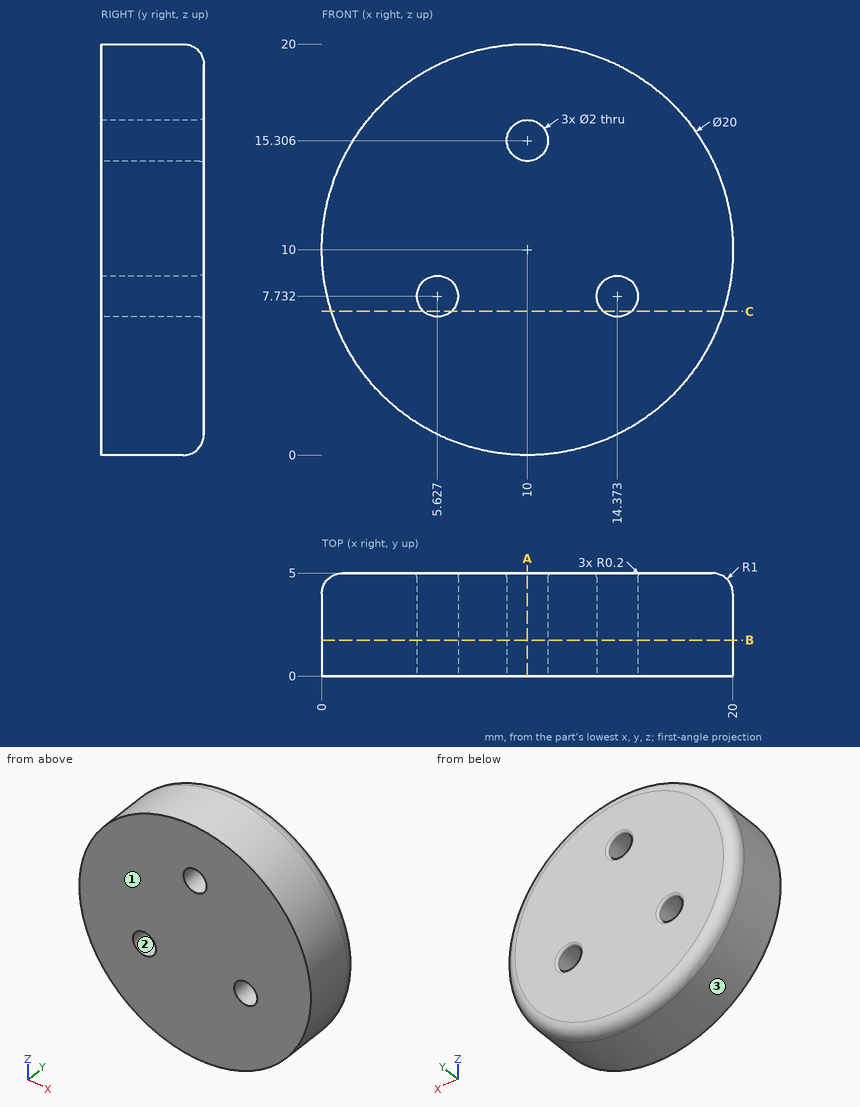
Job drawing, mm, ordinate dimensions from the low corner. One solid piece. Coordinates: 2 decimals unless noted, no trailing zeros. Order: outer loops, then holes, each group sorted by start corner. A loop starts at its lowest first (then second) coordinate and runs counter-clockwise, first axis right, second up. Notation, with made-up numbers: (1.5, -38) - (19.5, -38) arc R27 cw to (19.5, -7) - close; hole circle Ø8 at (-26, -5). An arc over 180 degrees is marked (long way). Write each question's results on one line, items separated by ' | '. Start each with the question number.
Item 1: Wall check: probe 1 along X at (y, z) = (4.5, 15.25); probe 2 along X at (y, z) = (0.6, 10); probe 3 along Z at (x, y) = (3, 1). Give the ranges that are in metal, low to high. Write a range as [from, to].
Item 2: Band-saw the part on B-B on y = 1.75. Write the cut outline in (x, z), and give its area (3 significant figures).
Item 3: Band-saw the part on A-A on x = 10. Write the cut outline in (y, z).
Item 4: Flat gauge pins, fed straight in: pin 1 (1 mm diameter, centred on y = 4, z = 2.5, fed in from +X); pin 2 (1 mm diameter, centred on x = 3.5, y = 3, fed in from +Z); pin 3 (2 mm diameter, centred on x = 2, y = 2, fed in from +Z). Where does each tip first touch, or does it go through?
Item 5: Band-saw the part on C-C on z = 7. State how many separate pieces and enclosed holes the cut face has.
Item 6: Mould opens along X. For the marked faces 1, 2 and 3 say: released by +X, released by -X, zero draft, split by the parting line, or undercut.
Numbers:
1) probe 1: [1.65, 9], [11, 18.35] | probe 2: [0, 20] | probe 3: [2.86, 17.14]
2) outline: circle Ø20 at (10, 10); hole circle Ø2 at (5.63, 7.73); hole circle Ø2 at (10, 15.31); hole circle Ø2 at (14.37, 7.73) | area: 305 mm^2
3) outline: (0, 0) - (4, 0) arc R1 ccw to (5, 1) - (5, 14.11) arc R0.2 ccw to (4.8, 14.31) - (0, 14.31) - close; (0, 16.31) - (4.8, 16.31) arc R0.2 ccw to (5, 16.51) - (5, 19) arc R1 ccw to (4, 20) - (0, 20) - close
4) pin 1: x = 17.14 | pin 2: z = 18 | pin 3: z = 17.14
5) separate pieces: 3 | enclosed holes: 0
6) face 1: zero draft | face 2: undercut | face 3: split by the parting line
